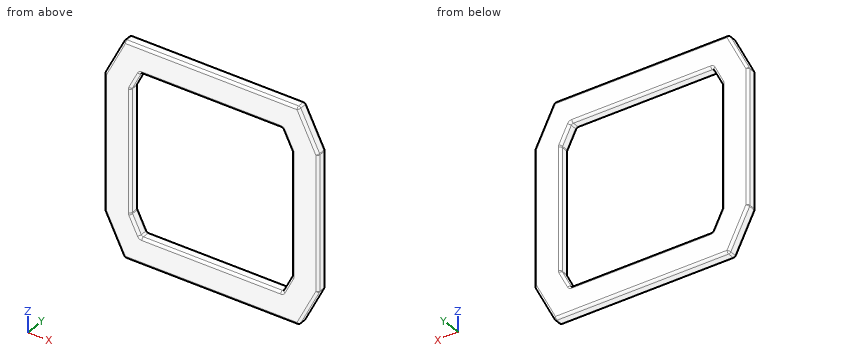
from build123d import *

# Parameters (mm, degrees)
BOSS_EXTRUDE1_DEPTH = 2.25
FILLET1_R           = 1


with BuildPart() as part:
    # Sketch1 → Boss-Extrude1 (new, symmetric)
    with BuildSketch(Plane(origin=(0, 0, 0), x_dir=(1, 0, 0), z_dir=(0, 1, 0))):
        Polygon((-36.298373876, -44.5), (36.298373876, -44.5), (44.5, -28.096747752), (44.5, 28.096747752), (36.298373876, 44.5), (-36.298373876, 44.5), (-44.5, 28.096747752), (-44.5, -28.096747752), align=None)
        Polygon((-29.5, -33.5), (29.5, -33.5), (33.5, -25.5), (33.5, 25.5), (29.5, 33.5), (-29.5, 33.5), (-33.5, 25.5), (-33.5, -25.5), align=None, mode=Mode.SUBTRACT)
    extrude(amount=BOSS_EXTRUDE1_DEPTH, both=True)

    # Fillet1
    fillet1_edges = [part.edges().sort_by_distance(p)[0] for p in [
        (44.5, -2.25, 0),
        (40.399186938, -2.25, 36.298373876),
        (0, -2.25, 44.5),
        (-40.399186938, -2.25, 36.298373876),
        (40.399186938, 2.25, 36.298373876),
        (-44.5, 0, 28.096747752),
        (-44.5, 0, -28.096747752),
        (-36.298373876, 0, -44.5),
        (36.298373876, 0, -44.5),
        (44.5, 0, -28.096747752),
        (44.5, 0, 28.096747752),
        (36.298373876, 0, 44.5),
        (-36.298373876, 0, 44.5),
        (44.5, 2.25, 0),
        (40.399186938, 2.25, -36.298373876),
        (0, 2.25, -44.5),
        (31.5, -2.25, -29.5),
        (33.5, 0, -25.5),
        (0, -2.25, -33.5),
        (29.5, 0, -33.5),
        (-31.5, -2.25, -29.5),
        (-29.5, 0, -33.5),
        (-33.5, -2.25, 0),
        (-40.399186938, 2.25, -36.298373876),
        (-33.5, 0, -25.5),
        (-31.5, -2.25, 29.5),
        (-33.5, 0, 25.5),
        (0, -2.25, 33.5),
        (-29.5, 0, 33.5),
        (31.5, -2.25, 29.5),
        (29.5, 0, 33.5),
        (33.5, -2.25, 0),
        (33.5, 0, 25.5),
        (31.5, 2.25, -29.5),
        (0, 2.25, -33.5),
        (-31.5, 2.25, -29.5),
        (-33.5, 2.25, 0),
        (-31.5, 2.25, 29.5),
        (0, 2.25, 33.5),
        (31.5, 2.25, 29.5),
        (-44.5, 2.25, 0),
        (33.5, 2.25, 0),
        (-40.399186938, 2.25, 36.298373876),
        (-44.5, -2.25, 0),
        (0, 2.25, 44.5),
        (-40.399186938, -2.25, -36.298373876),
        (0, -2.25, -44.5),
        (40.399186938, -2.25, -36.298373876),
    ]]
    fillet(fillet1_edges, radius=FILLET1_R)


solid = part.part
Check sheet for the modelled part. Datum: model origin and axes. Units: mm. Round coordinates to 2 decimals unless told otherwise and drop trailing zeros. Loops run counter-clockwise (first coordinate to the right, second up) from the corner with the lowest first, then second, coordinate; pieces in that order, holes last. Notation, with made-up numbers: (-24.5, 39.5) -> (-16.5, 39.5) arc R27 ccw to (-16.5, 61.5) -> close; hole circle Ø3 at (65.5, 87.5). An arc over 180 degrees is marked (long way). Put each result on its own line as item: value. Start each with the question number.
1. Scan lines: probe 1 along Z at (x, y) = (1.5, 0.1); probe 2 along X at (y, z) = (2.05, -17.5). Record each from-to range of solid material in increasing order.
2. Section check B-B (z = 16). Enter the section's corners in (x, y), plus the area to 3 significant figures.
3. Section check A-A (x = 22). Enter the section's corners in (y, z).
Findings:
1. probe 1: z = -44.5 to -33.5, 33.5 to 44.5
1. probe 2: x = -44.1 to -33.9, 33.9 to 44.1
2. outline: (-44.5, -1.25) arc R1 ccw to (-43.5, -2.25) -> (-34.5, -2.25) arc R1 ccw to (-33.5, -1.25) -> (-33.5, 1.25) arc R1 ccw to (-34.5, 2.25) -> (-43.5, 2.25) arc R1 ccw to (-44.5, 1.25) -> close; (33.5, -1.25) arc R1 ccw to (34.5, -2.25) -> (43.5, -2.25) arc R1 ccw to (44.5, -1.25) -> (44.5, 1.25) arc R1 ccw to (43.5, 2.25) -> (34.5, 2.25) arc R1 ccw to (33.5, 1.25) -> close
2. area: 97.3 mm^2
3. outline: (-2.25, -43.5) arc R1 ccw to (-1.25, -44.5) -> (1.25, -44.5) arc R1 ccw to (2.25, -43.5) -> (2.25, -34.5) arc R1 ccw to (1.25, -33.5) -> (-1.25, -33.5) arc R1 ccw to (-2.25, -34.5) -> close; (-2.25, 34.5) arc R1 ccw to (-1.25, 33.5) -> (1.25, 33.5) arc R1 ccw to (2.25, 34.5) -> (2.25, 43.5) arc R1 ccw to (1.25, 44.5) -> (-1.25, 44.5) arc R1 ccw to (-2.25, 43.5) -> close
